Model file for the job. Use its own axes, mm. A direction names the side the tool comes from. Coordinates: 2 decimals unless noted, no trailing zeros. Write each loop counter-clockwise with the first axis right and the second up, starting at its lowest first coordinate (ties: lowest second). Pieces come first, ordered by that corner, then holes.
Q1. Which spindle directions (+Z, -Z, +X, -X, +Y, -Y) get a long thin tool onto all of the face, cutting with end or side? Do faces 1 (the flat face through (-16, 0.3, 2.7)), 2 (the flat face through (-8, -0.1, 7.3)). Say none if no direction does.
Q2. Band-saw the part on C-C, the plane y = 10.75. Write the cut outline in (x, z), plus the area to 3 significant figures.
Q3. Band-saw the part on A-A, the plane y = 0. Write the cut outline in (x, z).
Q4. Drill centre lines: probe 1 along Y at (x, z) = (3.66, 5.75); probe 2 along Y at (x, z) = (0, 6); probe 3 along X at (y, z) = (-11, 2.5). Where is each one in solid material? Low to high.
Q5. Pull direction Y, two halves, no side cores. Call faces 3 (the flat face through (0, 9, 0)), 4 (the flat face through (15.5, -12.5, 4.9)), 5 (the flat face through (0, 13, 5)), 6 (the cylindrical face through (4.21, 11.26, 4.93)): released by +Y, released by -Y, zero draft, split by the parting line, or undercut.
Q6. Band-saw the part on D-D, the plane z = 8.5. Write the cut outline in (x, y), plus the area to 3 significant figures.
Q7. Band-saw the part on B-B, the plane x = 2. Write the cut outline in (y, z), plus the area to 3 significant figures.
from build123d import *

# Parameters (mm, degrees)
SKETCH_1_W          = 32
SKETCH_1_H          = 26
EXTRUDE_1_DEPTH     = 10
SKETCH_2_W          = 16
SKETCH_2_H          = 17
CUT_EXTRUDE_2_DEPTH = 23.912878475
FILLET_1_R          = 3
SKETCH_3_R          = 2
CUT_EXTRUDE_3_DEPTH = 36.958309193
CHAMFER_1_SIZE      = 1
SKETCH_4_R          = 0.75
CUT_EXTRUDE_1_DEPTH = 23.912878475


with BuildPart() as part:
    # Эскиз1 → Вытянуть1 (new body)
    with BuildSketch(Plane.XY):
        Rectangle(SKETCH_1_W, SKETCH_1_H)
    extrude(amount=EXTRUDE_1_DEPTH)

    # Эскиз2 → Вытянуть2 (cut, through all)
    with BuildSketch(Plane.XY.offset(10)):
        Rectangle(SKETCH_2_W, SKETCH_2_H)
    extrude(amount=-CUT_EXTRUDE_2_DEPTH, mode=Mode.SUBTRACT)

    # Скругление1
    fillet_1_edges = [part.edges().sort_by_distance(p)[0] for p in [
        (8, 8.5, 5),
        (8, -8.5, 5),
        (-8, -8.5, 5),
        (-8, 8.5, 5),
    ]]
    fillet(fillet_1_edges, radius=FILLET_1_R)

    # Эскиз3 → Вытянуть3 (cut, through all)
    with BuildSketch(Plane.ZY.offset(16)):
        with Locations((5, 0)):
            Circle(SKETCH_3_R)
    extrude(amount=-CUT_EXTRUDE_3_DEPTH, mode=Mode.SUBTRACT)

    # Фаска1
    chamfer_1_edges = [part.edges().sort_by_distance(p)[0] for p in [
        (16, -13, 5),
        (-16, -13, 5),
    ]]
    chamfer(chamfer_1_edges, length=CHAMFER_1_SIZE)

    # Эскиз4 → Вырез-Вытянуть1 (cut, through all)
    with BuildSketch(Plane(origin=(0, 0, 0), x_dir=(-1, 0, 0), z_dir=(0, 0, -1))):
        with Locations((-3.66, 10.75)):
            Circle(SKETCH_4_R)
        with Locations(Location((3.66, 10.75, 0), (0, 0, 180))):
            Circle(SKETCH_4_R)
        with Locations((3.66, -10.75)):
            Circle(SKETCH_4_R)
        with Locations(Location((-3.66, -10.75, 0), (0, 0, 180))):
            Circle(SKETCH_4_R)
    extrude(amount=-CUT_EXTRUDE_1_DEPTH, mode=Mode.SUBTRACT)


solid = part.part
Answer sheet:
1. face 1: +Z, -Z, -X, +Y, -Y
1. face 2: +Z, -Z
2. outline: (-16, 0) - (-4.41, 0) - (-4.41, 10) - (-16, 10) - close; (-2.91, 0) - (2.91, 0) - (2.91, 10) - (-2.91, 10) - close; (4.41, 0) - (16, 0) - (16, 10) - (4.41, 10) - close
2. area: 290 mm2
3. outline: (-16, 0) - (-8, 0) - (-8, 3) - (-16, 3) - close; (-16, 7) - (-8, 7) - (-8, 10) - (-16, 10) - close; (8, 0) - (16, 0) - (16, 3) - (8, 3) - close; (8, 7) - (16, 7) - (16, 10) - (8, 10) - close
4. probe 1: y = -13 to -11.5, -10 to -8.5, 8.5 to 10, 11.5 to 13
4. probe 2: y = -13 to -8.5, 8.5 to 13
4. probe 3: x = -16 to -4.37, -2.95 to 2.95, 4.37 to 16
5. face 3: zero draft
5. face 4: released by -Y
5. face 5: released by +Y
5. face 6: undercut
6. outline: (-16, -12) - (-15, -13) - (15, -13) - (16, -12) - (16, 13) - (-16, 13) - close; hole (-8, -5.5) arc R3 ccw to (-5, -8.5) - (5, -8.5) arc R3 ccw to (8, -5.5) - (8, 5.5) arc R3 ccw to (5, 8.5) - (-5, 8.5) arc R3 ccw to (-8, 5.5) - close; hole circle Ø1.5 at (-3.66, -10.75); hole circle Ø1.5 at (-3.66, 10.75); hole circle Ø1.5 at (3.66, -10.75); hole circle Ø1.5 at (3.66, 10.75)
6. area: 560 mm2
7. outline: (-13, 0) - (-8.5, 0) - (-8.5, 10) - (-13, 10) - close; (8.5, 0) - (13, 0) - (13, 10) - (8.5, 10) - close
7. area: 90.0 mm2
